Read the model definition and answer for the solid it produces. Units are mm, in the model's axes. Give positions to 0.01 mm unless a question says otherwise; leave off trailing zeros. Order: outer loops, then holes, each group sorted by start corner. A loop starts at its lowest first (then second) coordinate and runs counter-clockwise, first axis right, second up. Notation, with made-up numbers: (75, 38.5) - (134, 38.5) arc R18 cw to (134, 57.5) - close; hole circle Ø10 at (6, -14). An arc over 180 degrees is marked (long way). Answer as CSV lines item,"result". Start each with the question number.
from build123d import *

# Parameters (mm, degrees)
SKETCH3_R           = 50
BOSS_EXTRUDE2_DEPTH = 7


with BuildPart() as part:
    # Sketch3 → Boss-Extrude2 (new body)
    with BuildSketch(Plane(origin=(0, 0, 0), x_dir=(0, 0, -1), z_dir=(1, 0, 0))):
        Circle(SKETCH3_R)
        Polygon((0, 7.95), (-0.621944356, 5.917405277), (-1.652897942, 7.776273426), (-1.838651117, 5.658786272), (-3.233556312, 7.262686388), (-2.975, 5.152851153), (-4.672892756, 6.431685105), (-3.981327108, 4.421711712), (-5.908001363, 5.319588321), (-4.813651117, 3.497322251), (-6.88490196, 3.975), (-5.435595473, 2.420083026), (-7.560899305, 2.456685105), (-5.819978224, 1.23707456), (-7.906449068, 0.831001283), (-5.95, 0), (-7.906449068, -0.831001283), (-5.819978224, -1.23707456), (-7.560899305, -2.456685105), (-5.435595473, -2.420083026), (-6.88490196, -3.975), (-4.813651117, -3.497322251), (-5.908001363, -5.319588321), (-3.981327108, -4.421711712), (-4.672892756, -6.431685105), (-2.975, -5.152851153), (-3.233556312, -7.262686388), (-1.838651117, -5.658786272), (-1.652897942, -7.776273426), (-0.621944356, -5.917405277), (0, -7.95), (0.621944356, -5.917405277), (1.652897942, -7.776273426), (1.838651117, -5.658786272), (3.233556312, -7.262686388), (2.975, -5.152851153), (4.672892756, -6.431685105), (3.981327108, -4.421711712), (5.908001363, -5.319588321), (4.813651117, -3.497322251), (6.88490196, -3.975), (5.435595473, -2.420083026), (7.560899305, -2.456685105), (5.819978224, -1.23707456), (7.906449068, -0.831001283), (5.95, 0), (7.906449068, 0.831001283), (5.819978224, 1.23707456), (7.560899305, 2.456685105), (5.435595473, 2.420083026), (6.88490196, 3.975), (4.813651117, 3.497322251), (5.908001363, 5.319588321), (3.981327108, 4.421711712), (4.672892756, 6.431685105), (2.975, 5.152851153), (3.233556312, 7.262686388), (1.838651117, 5.658786272), (1.652897942, 7.776273426), (0.621944356, 5.917405277), align=None, mode=Mode.SUBTRACT)
        with BuildLine():
            Line((-1.092322441, 10.392753807), (-1.092322441, 47.987569554))
            ThreePointArc((-1.092322441, 47.987569554), (-33.941125497, 33.941125497), (-47.987569554, 1.092322441))
            Line((-47.987569554, 1.092322441), (-10.392753807, 1.092322441))
            ThreePointArc((-10.392753807, 1.092322441), (-7.389265863, 7.389265863), (-1.092322441, 10.392753807))
        make_face(mode=Mode.SUBTRACT)
        with BuildLine():
            Line((1.092322441, 10.392753807), (1.092322441, 47.987569554))
            ThreePointArc((1.092322441, 47.987569554), (33.941125497, 33.941125497), (47.987569554, 1.092322441))
            Line((47.987569554, 1.092322441), (10.392753807, 1.092322441))
            ThreePointArc((10.392753807, 1.092322441), (7.389265863, 7.389265863), (1.092322441, 10.392753807))
        make_face(mode=Mode.SUBTRACT)
        with BuildLine():
            Line((10.392753807, -1.092322441), (47.987569554, -1.092322441))
            ThreePointArc((47.987569554, -1.092322441), (33.941125497, -33.941125497), (1.092322441, -47.987569554))
            Line((1.092322441, -47.987569554), (1.092322441, -10.392753807))
            ThreePointArc((1.092322441, -10.392753807), (7.389265863, -7.389265863), (10.392753807, -1.092322441))
        make_face(mode=Mode.SUBTRACT)
        with BuildLine():
            Line((-1.092322441, -10.392753807), (-1.092322441, -47.987569554))
            ThreePointArc((-1.092322441, -47.987569554), (-33.941125497, -33.941125497), (-47.987569554, -1.092322441))
            Line((-47.987569554, -1.092322441), (-10.392753807, -1.092322441))
            ThreePointArc((-10.392753807, -1.092322441), (-7.389265863, -7.389265863), (-1.092322441, -10.392753807))
        make_face(mode=Mode.SUBTRACT)
    extrude(amount=BOSS_EXTRUDE2_DEPTH)


solid = part.part
(1) Flat-ended cylindrical pins translate along their axes: pin 1 Ø3.5 at (x, y) = (4, -30.5) entering from +Z; pin 2 Ø1 at (x, z) = (2, 5) entering from -Y; pin 3 Ø2 at (x, y) = (3, 20) entering from +Z. Find the tip coordinate at first contact, or state that the pin passes through.
(2) Straight lines are drawn through the part: line 1 (Z direction, x = 3, y = -10.5); line 2 (Z direction, x = 3, y = 15); line 3 (Y direction, x = 5, z = -21). For each, find the intervals that lie inside material, in ascending order. Write a range as [from, to].
(3) Determine the mould class of faces 1 (the cylindrical face through (3.45, 7.32, -7.46)), 2 (the flat face through (0, 8, 4)) for opening direction Y: released by +Y, released by -Y, zero draft, split by the parting line, or undercut.
(4) Section B-B, the plane z = -18 is taken. Write down the section's boundary in (x, y), and give its area (3 significant figures).
(5) Section A-A, the plane y = -43 is taken. Write down the section's boundary in (x, z).
(6) Section C-C, the plane x = 4.5 is taken. State how many separate pieces and enclosed holes the cut face has, and give its area (3 significant figures).
Checks:
1,pin 1,"stops at z = 40.91"
1,pin 2,"stops at y = -49.8"
1,pin 3,"stops at z = 46.25"
2,line 1,"z = [-48.89, -46.84], [-1.09, 1.09], [46.84, 48.89]"
2,line 2,"z = [-47.7, -45.6], [-1.09, 1.09], [45.6, 47.7]"
2,line 3,"y = [-45.38, -43.16], [-1.09, 1.09], [43.16, 45.38]"
3,face 1,"undercut"
3,face 2,"zero draft"
4,outline,"(0, -46.65) - (7, -46.65) - (7, -44.5) - (0, -44.5) - close; (0, -1.09) - (7, -1.09) - (7, 1.09) - (0, 1.09) - close; (0, 44.5) - (7, 44.5) - (7, 46.65) - (0, 46.65) - close"
4,area,"45.4 mm²"
5,outline,"(0, -25.51) - (7, -25.51) - (7, -21.33) - (0, -21.33) - close; (0, -1.09) - (7, -1.09) - (7, 1.09) - (0, 1.09) - close; (0, 21.33) - (7, 21.33) - (7, 25.51) - (0, 25.51) - close"
6,separate pieces,"1"
6,enclosed holes,"5"
6,area,"1,140 mm²"
